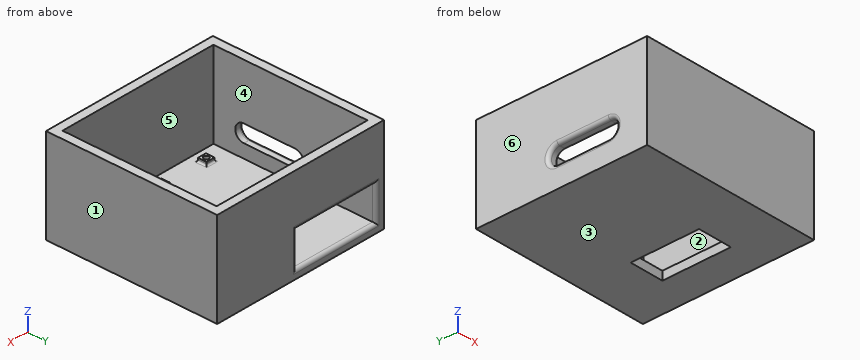
from build123d import *

# Parameters (mm, degrees)
SKETCH1_W           = 105
SKETCH1_H           = 100
SKETCH1_W_2         = 20
SKETCH1_H_2         = 40
BOSS_EXTRUDE1_DEPTH = 5
SKETCH2_W           = 105
SKETCH2_H           = 100
SKETCH2_W_2         = 95
SKETCH2_H_2         = 90
BOSS_EXTRUDE2_DEPTH = 50
SKETCH4_W           = 5
SKETCH4_H           = 5
SKETCH4_R           = 1.5
BOSS_EXTRUDE3_DEPTH = 2
FILLET1_R           = 1
SKETCH5_W           = 50
SKETCH5_H           = 20
CUT_EXTRUDE1_DEPTH  = 5
CUT_EXTRUDE2_DEPTH  = 5
FILLET2_R           = 2
FILLET3_R           = 2


with BuildPart() as part:
    # Sketch1 → Boss-Extrude1 (new body)
    with BuildSketch(Plane.XY):
        with Locations((-12.5, 20)):
            Rectangle(SKETCH1_W, SKETCH1_H)
        with Locations((10, 20)):
            Rectangle(SKETCH1_W_2, SKETCH1_H_2, mode=Mode.SUBTRACT)
    extrude(amount=BOSS_EXTRUDE1_DEPTH)

    # Sketch2 → Boss-Extrude2 (add)
    with BuildSketch(Plane.XY.offset(5)):
        with Locations((-12.5, 20)):
            Rectangle(SKETCH2_W, SKETCH2_H)
        with Locations((-12.5, 20)):
            Rectangle(SKETCH2_W_2, SKETCH2_H_2, mode=Mode.SUBTRACT)
    extrude(amount=BOSS_EXTRUDE2_DEPTH)

    # Sketch4 → Boss-Extrude3 (add)
    with BuildSketch(Plane.XY.offset(5)):
        with Locations((-52.46, 34.61)):
            Rectangle(SKETCH4_W, SKETCH4_H)
        with Locations((-52.46, 34.61)):
            Circle(SKETCH4_R, mode=Mode.SUBTRACT)
        with Locations((-4.2, 33.34)):
            Rectangle(SKETCH4_W, SKETCH4_H)
        with Locations((-4.2, 33.34)):
            Circle(SKETCH4_R, mode=Mode.SUBTRACT)
        with Locations((-47.38, -17.46)):
            Rectangle(SKETCH4_W, SKETCH4_H)
        with Locations((-47.38, -17.46)):
            Circle(SKETCH4_R, mode=Mode.SUBTRACT)
        with Locations((-19.46, -17.46)):
            Rectangle(SKETCH4_W, SKETCH4_H)
        with Locations((-19.46, -17.46)):
            Circle(SKETCH4_R, mode=Mode.SUBTRACT)
    extrude(amount=BOSS_EXTRUDE3_DEPTH)

    # Fillet1
    fillet1_edges = [part.edges().sort_by_distance(p)[0] for p in [
        (-49.96, 34.61, 5),
        (-52.46, 37.11, 5),
        (-54.96, 34.61, 5),
        (-52.46, 32.11, 5),
        (-1.7, 33.34, 5),
        (-4.2, 35.84, 5),
        (-6.7, 33.34, 5),
        (-4.2, 30.84, 5),
        (-44.88, -17.46, 5),
        (-47.38, -14.96, 5),
        (-49.88, -17.46, 5),
        (-47.38, -19.96, 5),
        (-16.96, -17.46, 5),
        (-19.46, -14.96, 5),
        (-21.96, -17.46, 5),
        (-19.46, -19.96, 5),
    ]]
    fillet(fillet1_edges, radius=FILLET1_R)

    # Sketch5 → Cut-Extrude1 (cut)
    with BuildSketch(Plane(origin=(0, 70, 0), x_dir=(1, 0, 0), z_dir=(0, 1, 0))):
        with Locations((-35, -15)):
            Rectangle(SKETCH5_W, SKETCH5_H)
    extrude(amount=-CUT_EXTRUDE1_DEPTH, mode=Mode.SUBTRACT)

    # Sketch6 → Cut-Extrude2 (cut)
    with BuildSketch(Plane.ZY.offset(65)):
        with BuildLine():
            Line((22.805324428, 22.755889518), (22.805324428, -7.244110482))
            ThreePointArc((22.805324428, -7.244110482), (17.805324428, -12.244110482), (12.805324428, -7.244110482))
            Line((12.805324428, -7.244110482), (12.805324428, 22.755889518))
            ThreePointArc((12.805324428, 22.755889518), (17.805324428, 27.755889518), (22.805324428, 22.755889518))
        make_face()
    extrude(amount=-CUT_EXTRUDE2_DEPTH, mode=Mode.SUBTRACT)

    # Fillet2
    fillet2_edges = [part.edges().sort_by_distance(p)[0] for p in [
        (-65, 27.755889518, 17.805324428),
        (-65, 7.755889518, 12.805324428),
        (-65, -12.244110482, 17.805324428),
        (-65, 7.755889518, 22.805324428),
    ]]
    fillet(fillet2_edges, radius=FILLET2_R)

    # Fillet3
    fillet3_edges = [part.edges().sort_by_distance(p)[0] for p in [
        (-60, 70, 15),
        (-35, 70, 25),
        (-10, 70, 15),
        (-35, 70, 5),
    ]]
    fillet(fillet3_edges, radius=FILLET3_R)


solid = part.part
Input: part model. Units: mm. Frame: model coordinates. Face numbers are marked on the shaded views. A direction names the side the tool comes from. Give positions to 0.01 mm unless a question says otherwise; leave off trailing zeros. Write each loop counter-clockwise with the first axis right and the second up, starting at its lowest first coordinate (ties: lowest second). Pieces come first, ordered by that corner, then holes. Notation, with made-up numbers: (-30.5, 73) -> (-23.5, 73) arc R34 ccw to (-23.5, 110) -> close; hole circle Ø5 at (30, 3). An arc over 180 degrees is marked (long way). Use one line per item in the form item = value. Start each with the question number.
1) Section query A-A on x = -19.46. Return the cut outline in (y, z).
2) Section query C-C on y = -17.46. Return the cut outline in (x, z), then the cut area to 3 significant figures.
3) Pin query (flat end, axial travel): pin 1 (3 mm diameter, centred on x = -37.5, z = 7, fed in from +Y); pin 2 (6 mm diameter, centred on y = 14.5, z = 19.5, fed in from -X); pin 3 (1.5 mm diameter, centred on x = 19, y = -15.5, fed in from +Z). Return the tip coordinate at first contact, or that it passes through.
4) Draft query along X for the marked faces 3, 4, 5 and 6. Return one class per face: pulls with the +X half, pulls with the -X half, needs draft (parallel to the pull), parting line crosses it, or undercut.
5) Section query D-D on x = 30. Return the cut outline in (y, z).
6) Set-up query: the marked faces 1 and 2. Return all of +Z, -Z, +X, -X, +Y, -Y with unobstructed straight access to the full face (end or side cutting, diameter ignored); none if empty.
7) Section query B-B on z = 46. Return the cut outline in (x, y), then the cut area to 3 significant figures.
8) Ray query, probe 1 along Y at (x, z) = (-52.46, 5.75); probe 2 along Y at (x, z) = (-7, 11); probe 3 along Y at (x, z) = (-50.5, 6.5). Return the intervals inside material, ascending. Write a range as from..to.
Outcome:
q1.outline = (-30, 0) -> (70, 0) -> (70, 3) arc R2 ccw to (68, 5) -> (-13.96, 5) arc R1 cw to (-14.96, 6) -> (-14.96, 7) -> (-15.96, 7) -> (-15.96, 5) -> (-18.96, 5) -> (-18.96, 7) -> (-19.96, 7) -> (-19.96, 6) arc R1 cw to (-20.96, 5) -> (-25, 5) -> (-25, 55) -> (-30, 55) -> close; (65, 25) -> (68, 25) arc R2 ccw to (70, 27) -> (70, 55) -> (65, 55) -> close
q2.outline = (-65, 0) -> (40, 0) -> (40, 55) -> (35, 55) -> (35, 5) -> (-15.96, 5) arc R1 cw to (-16.96, 6) -> (-16.96, 7) -> (-17.96, 7) -> (-17.96, 5) -> (-20.96, 5) -> (-20.96, 7) -> (-21.96, 7) -> (-21.96, 6) arc R1 cw to (-22.96, 5) -> (-43.88, 5) arc R1 cw to (-44.88, 6) -> (-44.88, 7) -> (-45.88, 7) -> (-45.88, 5) -> (-48.88, 5) -> (-48.88, 7) -> (-49.88, 7) -> (-49.88, 6) arc R1 cw to (-50.88, 5) -> (-60, 5) -> (-60, 55) -> (-65, 55) -> close
q2.area = 1,030 mm^2
q3.pin_1 = -25
q3.pin_2 = 35
q3.pin_3 = 5
q4.face_3 = needs draft
q4.face_4 = undercut
q4.face_5 = undercut
q4.face_6 = pulls with the -X half
q5.outline = (-30, 0) -> (70, 0) -> (70, 55) -> (65, 55) -> (65, 5) -> (-25, 5) -> (-25, 55) -> (-30, 55) -> close
q6.face_1 = +Z, -Z, +X, +Y, -Y
q6.face_2 = +Z
q7.outline = (-65, -30) -> (40, -30) -> (40, 70) -> (-65, 70) -> close; hole (-60, -25) -> (35, -25) -> (35, 65) -> (-60, 65) -> close
q7.area = 1,950 mm^2
q8.probe_1 = -30..-25, 32.08..33.11, 36.11..37.14
q8.probe_2 = -30..-25, 65..70
q8.probe_3 = -30..-25, 32.11..37.11
